```python
from build123d import *

# Parameters (mm, degrees)
SKETCH1_W           = 112
SKETCH1_H           = 120
BOSS_EXTRUDE1_DEPTH = 3
SKETCH2_R           = 9.25
CUT_EXTRUDE1_DEPTH  = 10
CUT_EXTRUDE2_DEPTH  = 10


with BuildPart() as part:
    # Sketch1 → Boss-Extrude1 (new body)
    with BuildSketch(Plane(origin=(0, 0, 0), x_dir=(1, 0, 0), z_dir=(0, 1, 0))):
        Rectangle(SKETCH1_W, SKETCH1_H)
    extrude(amount=BOSS_EXTRUDE1_DEPTH)

    # Sketch2 → Cut-Extrude1 (cut)
    with BuildSketch(Plane(origin=(0, 3, 0), x_dir=(1, 0, 0), z_dir=(0, 1, 0))):
        Circle(SKETCH2_R)
    extrude(amount=-CUT_EXTRUDE1_DEPTH, mode=Mode.SUBTRACT)

    # Sketch3 → Cut-Extrude2 (cut)
    with BuildSketch(Plane(origin=(0, 3, 0), x_dir=(1, 0, 0), z_dir=(0, 1, 0))):
        with BuildLine():
            Line((-3, -60), (-3, -47))
            ThreePointArc((-3, -47), (0, -44), (3, -47))
            Line((3, -47), (3, -60))
            Line((3, -60), (-3, -60))
        make_face()
        with BuildLine():
            Line((-3, 60), (3, 60))
            Line((3, 60), (3, 47))
            ThreePointArc((3, 47), (0, 44), (-3, 47))
            Line((-3, 47), (-3, 60))
        make_face()
        with BuildLine():
            Line((56, 3), (43, 3))
            ThreePointArc((43, 3), (40, 0), (43, -3))
            Line((43, -3), (56, -3))
            Line((56, -3), (56, 3))
        make_face()
        with BuildLine():
            Line((-43, -3), (-56, -3))
            Line((-56, -3), (-56, 3))
            Line((-56, 3), (-43, 3))
            ThreePointArc((-43, 3), (-40, 0), (-43, -3))
        make_face()
    extrude(amount=-CUT_EXTRUDE2_DEPTH, mode=Mode.SUBTRACT)


solid = part.part
```
Could you check a few things on this model? Use its own coordinates, in mm. A direction names the side the tool comes from. Round coordinates to 2 decimals unless told otherwise and drop trailing zeros. Write each loop counter-clockwise with the first axis right and the second up, starting at its lowest first coordinate (ties: lowest second). Pieces come first, ordered by that corner, then holes. Notation, with made-up numbers: M 53,38 L 76,38 A30 ccw 76,66 Z; hole C 61,74 d1. An arc over 180 degrees is marked long. Write each question's results on one line, items separated by ' | '. Start each with the question number.
1. Thinking about a two-plate mould opening in X: for faces 1 (the face through (-3, 2, 54)), 2 (the face through (-56, 1, -31)), 3 (the face through (3, 2, 53)), 4 (the face through (40, 2, 0)), which applies, +X half, -X half, draft (parallel to the pull), parting line (faces both ways), or undercut?
2. Imagine slicing it at B-B on y = 1.7. List the corners of the cut face in (x, z) for me.
3. Imagine slicing it at A-A on x = 0. List the corners of the cut face in (y, z) for me.
4. On a 3-axis mill with a long thin cutter (end or side, diameter ignored), from which of +Z, -Z, +X, -X, +Y, -Y can I reach the whole of each face in a straight line? I mean faces 5 (the face through (-2.01, 1.52, 9.03)), 6 (the face through (50, 2, -3)), 7 (the face through (-49, 2, 3)). Say none if no direction works.
5. I need wall thicknesses on L1, parallel to X at y = 1.7, z = 0; L2, parallel to Z at x = 0, y = 0.7; L3, parallel to X at y = 1.9, z = 54. Which ranges of each line are inside material? Lowest first, please. Write a range as from..to.
6. Imagine slicing it at C-C on z = -45.5. List the corners of the cut face in (x, y) for me, and give its area (3 significant figures).
Result sheet:
1) face 1: undercut | face 2: -X half | face 3: undercut | face 4: +X half
2) outline: M -56,-60 L -3,-60 L -3,-47 A3 cw 3,-47 L 3,-60 L 56,-60 L 56,-3 L 43,-3 A3 cw 43,3 L 56,3 L 56,60 L 3,60 L 3,47 A3 cw -3,47 L -3,60 L -56,60 L -56,3 L -43,3 A3 cw -43,-3 L -56,-3 Z; hole C 0,0 d18.5
3) outline: M 0,-44 L 3,-44 L 3,-9.25 L 0,-9.25 Z; M 0,9.25 L 3,9.25 L 3,44 L 0,44 Z
4) face 5: +Y, -Y | face 6: +X, +Y, -Y | face 7: -X, +Y, -Y
5) L1: x = -40..-9.25, 9.25..40 | L2: z = -44..-9.25, 9.25..44 | L3: x = -56..-3, 3..56
6) outline: M -56,0 L -2.6,0 L -2.6,3 L -56,3 Z; M 2.6,0 L 56,0 L 56,3 L 2.6,3 Z | area: 320 mm^2
